from build123d import *

# Parameters (mm, degrees)
F0_W      = 60
F0_H      = 50
F1_DEPTH  = 60
F2_W      = 10
F2_H      = 50
F3_DEPTH  = 40
F5_DEPTH  = 40
F6_W      = 10
F6_H      = 50
F7_DEPTH  = 40
F14_DEPTH = 10
F16_DEPTH = 50.001
F20_DEPTH = 25


with BuildPart() as f1:
    # F0 (on Top) → F1 (new body)
    with BuildSketch(Plane.XY):
        with Locations((30, 25)):
            Rectangle(F0_W, F0_H)
    extrude(amount=F1_DEPTH)

    # F2 (on face) → F3 (cut)
    with BuildSketch(Plane.XY.offset(60)):
        with Locations((5, 25)):
            Rectangle(F2_W, F2_H)
    extrude(amount=-F3_DEPTH, mode=Mode.SUBTRACT)

    # F4 (on face) → F5 (cut)
    with BuildSketch(Plane.XY.offset(60)):
        Polygon((20, 50), (10, 50), (10, 40), align=None)
    extrude(amount=-F5_DEPTH, mode=Mode.SUBTRACT)

    # F6 (on face) → F7 (cut)
    with BuildSketch(Plane.XY.offset(60)):
        with Locations((55, 25)):
            Rectangle(F6_W, F6_H)
    extrude(amount=-F7_DEPTH, mode=Mode.SUBTRACT)

    # F12: sweep along a path in F11
    with BuildLine(Plane.YZ.offset(30)) as f12_path:
        Line((0, 45), (50, 60))
    # F9 (on face) → F12 (sweep, cut)
    with BuildSketch(Plane.XZ):
        Polygon((50, 60), (10, 60), (30, 45), align=None)
    sweep(path=f12_path.line, mode=Mode.SUBTRACT)

    # F13 (on face) → F14 (cut)
    with BuildSketch(Plane(origin=(0, 0, 0), x_dir=(1, 0, 0), z_dir=(0, 0, -1))):
        Polygon((30, 0), (0, 0), (30, -50), (60, -50), align=None)
    extrude(amount=-F14_DEPTH, mode=Mode.SUBTRACT)

    # F15 (on face) → F16 (cut, through all)
    with BuildSketch(Plane.YZ.offset(50)):
        Polygon((0, 35), (0, 20), (8.6602540378, 20), align=None)
    extrude(amount=-F16_DEPTH, mode=Mode.SUBTRACT)

    # F19 (on 3pt) → F20 (cut)
    with BuildSketch(Plane(origin=(56.7375886525, 22.695035461, 28.3687943262), x_dir=(-0.3012974309, 0.9415544714, -0.1506487154), z_dir=(0.8421519211, 0.3368607684, 0.4210759605))):
        Polygon((28.9998777205, 40.249223595), (-24.103794469, 31.304951685), (28.9998777205, -4.472135955), align=None)
    extrude(amount=F20_DEPTH, mode=Mode.SUBTRACT)


solid = f1.part
Check sheet for the modelled part. Datum: model origin and axes. Units: mm. A direction names the side the tool comes from. Give positions to 0.01 mm unless a question says otherwise; leave off trailing zeros. Write each loop counter-clockwise with the first axis right and the second up, starting at its lowest first coordinate (ties: lowest second). Pieces come first, ordered by that corner, then holes. Notation, with made-up numbers: (21.25, -22) -> (55.25, -22) arc R23 ccw to (55.25, 6) -> close; hole circle Ø5 at (-10.75, -12.75). An arc over 180 degrees is marked (long way). Use one line per item in the form item = value. Start each with the question number.
1. Section check C-C (y = 4). Record the cut outline in (x, z), and give its area (3 significant figures).
2. Mould release check, pull along X, two halves, no side actions. Record for faces 5 (the flat face through (0, 25, 10)), 6 (the flat face through (45, 25, 5)), 7 (the flat face through (30, 50, 23)), 8 (the flat face through (15, 25, 5)): pulls with the +X half, pulls with the -X half, needs draft (parallel to the pull), parting line crosses it, or undercut.
3. Go/stop test with flat-tipped pins: P1, Ø4, axis at x = 36.5, y = 33, coming from the +Z side; P2, Ø8, axis at x = 42.5, y = 35, coming from the +Z side; P3, Ø6, axis at x = 29, y = 10, coming from the +Z side; P4, Ø1, axis at x = 25, y = 16, coming from the -Z side. Record where each tip stops, or that it passes through.
4. Thickness scan on line 1 along Z through (x, y) = (54, 5); line 2 along X through (y, z) = (19, 57.5); line 3 along X through (y, z) = (10, 52.5). Record the ranges inside material, lowest first. Write a range as from..to.
5. Section check D-D (z = 51). Record the cut outline in (x, y).
6. Access from +Z, -Z, +X, -X, +Y, -Y to the whole of each face (thin tool, end or side, straight path). Record for faces 1 (the flat face through (50, 14, 31)), 2 (the flat face through (30.28, 4.39, 27.4)), 3 (the flat face through (37.01, 19.794, 56.196)), 4 (the flat face through (30, 25, 10)).
7. Section check A-A (z = 6). Record the cut outline in (x, y), and give its area (3 significant figures).
8. Section check B-B (y = 13.5). Record the cut outline in (x, z), and give its area (3 significant figures).
Conclusion:
q1.outline = (0, 0) -> (2.4, 0) -> (2.4, 10) -> (32.4, 10) -> (32.4, 0) -> (60, 0) -> (60, 20) -> (0, 20) -> close; (10, 28.07) -> (50, 28.07) -> (50, 56.8) -> (48.4, 60) -> (30, 46.2) -> (11.6, 60) -> (10, 60) -> close
q1.area = 1,920 mm²
q2.face_5 = pulls with the -X half
q2.face_6 = undercut
q2.face_7 = needs draft
q2.face_8 = undercut
q3.P1 = 60
q3.P2 = 55.62
q3.P3 = 51.17
q3.P4 = 10
q4.line_1 = 0..20
q4.line_2 = 10..20.93, 39.07..43.65
q4.line_3 = 10..24, 36..49.75
q5.outline = (10, 0) -> (22, 0) -> (30, 20) -> (38, 0) -> (50, 0) -> (50, 11.25) -> (34.5, 50) -> (20, 50) -> (10, 40) -> close
q6.face_1 = +Z, +X, +Y, -Y
q6.face_2 = +X, -X, -Y
q6.face_3 = +Z, -Y
q6.face_4 = -Z
q7.outline = (0, 0) -> (30, 50) -> (0, 50) -> close; (30, 0) -> (60, 0) -> (60, 50) -> close
q7.area = 1,500 mm²
q8.outline = (0, 0) -> (8.1, 0) -> (8.1, 10) -> (38.1, 10) -> (38.1, 0) -> (60, 0) -> (60, 20) -> (50, 20) -> (50, 49.2) -> (44.6, 60) -> (30, 49.05) -> (15.4, 60) -> (10, 60) -> (10, 20) -> (0, 20) -> close
q8.area = 2,310 mm²
